Work out the finished part from the listing and answer in its coordinate system (mm). Give positions to 0.01 mm unless a question says otherwise; leave off trailing zeros. Loops run counter-clockwise (first coordinate to the right, second up) from the corner with the lowest first, then second, coordinate; pieces in that order, holes last.
```python
from build123d import *

# Parameters (mm, degrees)
CYLINDER_R     = 20
CYLINDER_DEPTH = 3
BOX002_W       = 170
BOX002_H       = 110
BOX002_DEPTH   = 3


with BuildPart() as cilindro:
    # Cylinder → Cylinder (new body)
    with BuildSketch(Plane(origin=(80, 0, 0), x_dir=(1, 0, 0), z_dir=(0, 0, 1))):
        Circle(CYLINDER_R)
    extrude(amount=CYLINDER_DEPTH)


with BuildPart() as obj1:
    # Box002 → Box002 (new body)
    with BuildSketch(Plane.XY):
        with Locations((85, 55)):
            Rectangle(BOX002_W, BOX002_H)
    extrude(amount=BOX002_DEPTH)

    # Fusion: union Cilindro
    add(cilindro.part)


with BuildPart() as obj1_1:
    # Fusion placement: moved
    add(obj1.part.moved(Location((5, -30, 5))))


solid = obj1_1.part
```
Q1. Consider line 1 along Y through (x, z) = (35, 7.2); line 2 along Y through (x, z) = (86, 5.25); line 3 along X through (y, z) = (-42, 6.05). Determine where each line is inside the solid, lowest interval first.
Q2. Section C-C on y = -37 is taken. Give the vertices of the cut face in (x, z) (3 decimals), plus the area to 3 significant figures.
Q3. Given pin 1 (1.5 mm diameter, centred on x = 36.5, z = 6, fed in from -Y), flat-ended and moving along its own axis, determine where the tip first touches the part or whether it passes through.
Q4. Section A-A on z = 5.7 is taken. Give the vertices of the cut face in (x, y), plus the area to 3 significant figures.
Q5. Section B-B on x = 121.5 is taken. Give the vertices of the cut face in (y, z), plus the area to 3 significant figures.
Check result:
1. line 1: y = -30 to 80
1. line 2: y = -49.97 to 80
1. line 3: x = 69 to 101
2. outline: (66.265, 5) - (103.735, 5) - (103.735, 8) - (66.265, 8) - close
2. area: 112 mm2
3. pin 1: stops at y = -30
4. outline: (5, -30) - (65, -30) arc R20 ccw to (105, -30) - (175, -30) - (175, 80) - (5, 80) - close
4. area: 19,300 mm2
5. outline: (-30, 5) - (80, 5) - (80, 8) - (-30, 8) - close
5. area: 330 mm2
